```python
from build123d import *

# Parameters (mm, degrees)
F0_R      = 21.59
F1_DEPTH  = 482.6
F2_R      = 6.35
F3_R      = 6.35
F1_FACE_R = 15.24
F4_DEPTH  = 469.9


with BuildPart() as f1:
    # F0 (on Top) → F1 (new body)
    with BuildSketch(Plane.XY):
        Circle(F0_R)
    extrude(amount=F1_DEPTH)

    # F2
    f2_edges = [f1.edges().sort_by_distance(p)[0] for p in [
        (-21.59, 0, 0),
    ]]
    fillet(f2_edges, radius=F2_R)

    # F3
    f3_edges = [f1.edges().sort_by_distance(p)[0] for p in [
        (-21.59, 0, 482.6),
    ]]
    fillet(f3_edges, radius=F3_R)

    # F1_face (on face) → F4 (cut)
    with BuildSketch(Plane(origin=(0, 0, 0), x_dir=(1, 0, 0), z_dir=(0, 0, -1))):
        Circle(F1_FACE_R)
    extrude(amount=-F4_DEPTH, mode=Mode.SUBTRACT)


solid = f1.part
```
Work out the finished part from the listing and answer in its coordinate system (mm). Coordinates: 2 decimals unless noted, no trailing zeros. Write each loop counter-clockwise with the first axis right and the second up, starting at its lowest first coordinate (ties: lowest second). Pieces come first, ordered by that corner, then holes. Notation, with made-up numbers: (60.25, -35.5) - (103.25, -35.5) arc R15 ccw to (103.25, -27.5) - close; hole circle Ø6 at (80, 48). An arc over 180 degrees is marked (long way). Answer as a JSON object with one key per item and string values.
Q1. Find section A-A (x = 0). Write down the section's boundary in (y, z).
Results list:
{"outline": "(-21.59, 6.35) arc R6.35 ccw to (-15.24, 0) - (-15.24, 469.9) - (15.24, 469.9) - (15.24, 0) arc R6.35 ccw to (21.59, 6.35) - (21.59, 476.25) arc R6.35 ccw to (15.24, 482.6) - (-15.24, 482.6) arc R6.35 ccw to (-21.59, 476.25) - close"}
Q2. Given pin 1 Ø12 at (x, y) = (-14, 7) entering from +Z; pin 2 Ø10 at (x, z) = (-14.5, 230.5) entering from -Y; pin 3 Ø10 at (x, z) = (-9, 130) entering from +Y; pin 4 Ø1.5 at (y, z) = (12.5, 63) entering from -X, each flat-ended and moving along its own axis, determine where each tip first touches the part or whether it passes through.
Results list:
{"pin 1": "stops at z = 482.6", "pin 2": "stops at y = -19.39", "pin 3": "stops at y = 21.22", "pin 4": "stops at x = -18.11"}
Q3. For a pull along X with two mould halves and no side action, classify faces 1 (the cylindrical face through (-15.913, 14.592, 238.011)), 2 (the flat face through (0, 0, 482.6)), 3 (the flat face through (0, 0, 469.9)) as pulls with the +X half, pulls with the -X half, needs draft (parallel to the pull), parting line crosses it, or undercut.
Results list:
{"face 1": "parting line crosses it", "face 2": "needs draft", "face 3": "undercut"}
Q4. Find section C-C (z = 345). Write down the section's boundary in (x, y), plus the area to 3 significant figures.
Results list:
{"outline": "circle Ø43.18 at (0, 0); hole circle Ø30.48 at (0, 0)", "area": "735 mm^2"}
Q5. Consider L1, parallel to Y at x = 0, z = 315; L2, parallel to Y at x = 3, z = 452; L3, parallel to Z at x = 1, y = 5. Determine where each line is inside the solid, lowest interval first. Write a range as from..to.
Results list:
{"L1": "y = -21.59..-15.24, 15.24..21.59", "L2": "y = -21.38..-14.94, 14.94..21.38", "L3": "z = 469.9..482.6"}
